Verification items for the finished model (mm, model axes). Face numbers are marked on the shaded views. A direction names the side the tool comes from. Give positions to 0.01 mm unless a question says otherwise; leave off trailing zeros. Write each loop counter-clockwise with the first axis right and the second up, starting at its lowest first coordinate (ties: lowest second). Pieces come first, ordered by that corner, then holes. Notation, with made-up numbers: (76.5, -14) - (96.5, -14) arc R25 cw to (96.5, 24) - close; hole circle Ø10 at (10, 8). An arc over 180 degrees is marked (long way). Answer as a JSON object with one key per item and string values. Group by question number.
Item 1: Sectioned sample at A-A, the plane x = 0.4. Record the boundary of the cut face in (y, z), and give its area (3 significant figures).
Item 2: Sectioned sample at B-B, the plane y = 2.75. Record the boundary of the cut face in (x, z).
Item 3: Tool access check on the marked faces 1 and 2. Record the directions out of +Z, -Z, +X, -X, +Y, -Y that give a thin tool (end or side, any length) a straight path to the whole face; none if there is none.
Item 4: Sectioned sample at D-D, the plane z = -7.5. Record the boundary of the cut face in (x, y).
Item 5: Go/stop test with a flat-tipped pin: pin 1 (0.5 mm diameter, centred on x = 0, z = -3, fed in from -Y). Record where the tip stops, or that it passes through.
Item 6: Sectioned sample at C-C, the plane x = -0.05. Record the boundary of the cut face in (y, z).
Item 7: Scan lines: line 1 along Z through (x, y) = (0.1, 5.25); line 2 along Y through (x, z) = (0.35, -6); line 3 along Z through (x, y) = (-0.4, 7.5). Record each from-to range of solid material in increasing order. Write a range as [from, to].
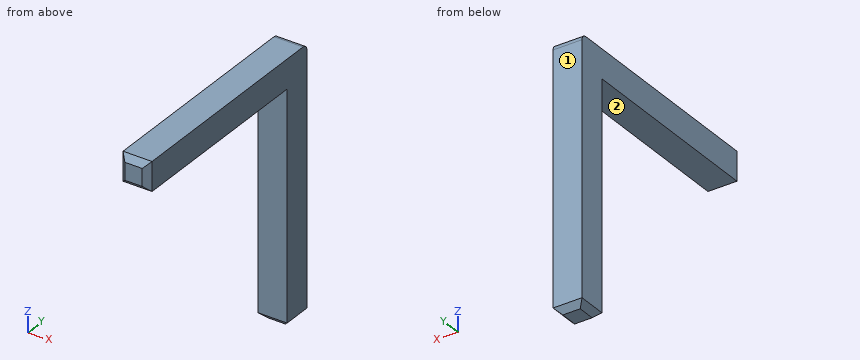
```python
from build123d import *

# Parameters (mm, degrees)
SKETCH2_W           = 1
SKETCH2_H           = 1
BOSS_EXTRUDE1_DEPTH = 8
SKETCH3_W           = 1
SKETCH3_H           = 1
BOSS_EXTRUDE2_DEPTH = 8
FILLET1_R           = 0.2
CHAMFER1_SIZE       = 0.2
CHAMFER2_SIZE       = 0.2


with BuildPart() as part:
    # Sketch2 → Boss-Extrude1 (new body)
    with BuildSketch(Plane(origin=(0, 0, 0), x_dir=(1, 0, 0), z_dir=(0, 1, 0))):
        Rectangle(SKETCH2_W, SKETCH2_H)
    extrude(amount=BOSS_EXTRUDE1_DEPTH)

    # Sketch3 → Boss-Extrude2 (add)
    with BuildSketch(Plane(origin=(0, 0, -0.5), x_dir=(-1, 0, 0), z_dir=(0, 0, -1))):
        with Locations((0, 7.5)):
            Rectangle(SKETCH3_W, SKETCH3_H)
    extrude(amount=BOSS_EXTRUDE2_DEPTH)

    # Fillet1
    fillet1_edges = [part.edges().sort_by_distance(p)[0] for p in [
        (0, 8, 0.5),
    ]]
    fillet(fillet1_edges, radius=FILLET1_R)

    # Chamfer1
    chamfer1_edges = [part.edges().sort_by_distance(p)[0] for p in [
        (0.5, 7.5, -8.5),
        (0, 7, -8.5),
        (-0.5, 7.5, -8.5),
        (0, 8, -8.5),
    ]]
    chamfer(chamfer1_edges, length=CHAMFER1_SIZE)

    # Chamfer2
    chamfer2_edges = [part.edges().sort_by_distance(p)[0] for p in [
        (-0.5, 0, 0),
        (0, 0, -0.5),
        (0.5, 0, 0),
        (0, 0, 0.5),
    ]]
    chamfer(chamfer2_edges, length=CHAMFER2_SIZE)


solid = part.part
```
Geometry check:
{
 "1": {"outline": "(0.1, -0.4) - (0.2, -0.5) - (7, -0.5) - (7, -8.3) - (7.1, -8.4) - (7.9, -8.4) - (8, -8.3) - (8, 0.3) arc R0.2 ccw to (7.8, 0.5) - (0.2, 0.5) - (0.1, 0.4) - close", "area": "15.8 mm^2"},
 "2": {"outline": "(-0.5, -0.5) - (0.5, -0.5) - (0.5, 0.5) - (-0.5, 0.5) - close"},
 "3": {"face 1": "+Z, -Z, +X, -X, +Y", "face 2": "-Z, +X, -X, -Y"},
 "4": {"outline": "(-0.5, 7) - (0.5, 7) - (0.5, 8) - (-0.5, 8) - close"},
 "5": {"pin 1": "y = 7"},
 "6": {"outline": "(0, -0.3) - (0.2, -0.5) - (7, -0.5) - (7, -8.3) - (7.2, -8.5) - (7.8, -8.5) - (8, -8.3) - (8, 0.3) arc R0.2 ccw to (7.8, 0.5) - (0.2, 0.5) - (0, 0.3) - close"},
 "7": {"line 1": "[-0.5, 0.5]", "line 2": "[7, 8]", "line 3": "[-8.4, 0.5]"}
}
